The listing builds one solid part. Answer for the finished solid, in the listing's coordinates (mm). A direction names the side the tool comes from. Coordinates: 2 decimals unless noted, no trailing zeros. Loops run counter-clockwise (first coordinate to the right, second up) from the corner with the lowest first, then second, coordinate; pieces in that order, holes last. Notation, with made-up numbers: (-3, 0.5) - (45, 0.5) arc R30 cw to (45, 38.5) - close; hole circle Ø10 at (39.25, -3). An arc over 180 degrees is marked (long way). Return JSON: item names as keys, results as strings. Group by question number.
1. This flat-tipped pin is pushed along its axis until it touches: P1, Ø1, axis at y = -5.5, z = 13, coming from the -X side. Where does it stop, or does it pass through?
2. Which of the six approach directions +Z, -Z, +X, -X, +Y, -Y give full straight-line access (tool end or side, diameter ignored) to faces 4 (the face through (0, 2, 15)), 5 (the face through (17.26, 0.5, 15.18))?
3. Find the intervals of material crossed by line 1 along Z through (x, y) = (29.25, 4); line 2 along Z through (x, y) = (29, -2); line 3 along Z through (x, y) = (29.25, -2.5), in increasing order.
4. Section B-B (z = 2.75) is taken. Write down the section's boundary in (x, y).
5. Section A-A (x = 29.25) is taken. Write down the section's boundary in (y, z), and give its area (3 significant figures).
6. Section D-D (x = 10.5) is taken. Write down the section's boundary in (y, z).
7. The mould has two halves that part along Z. Classify faces 1 (the face through (27.736, 0.098, 3.227)), 2 (the face through (20, 0, 30)), 3 (the face through (40, 0, 15)): pulls with the +Z half, pulls with the -Z half, needs draft (parallel to the pull), parting line crosses it, or undercut.
Autodesk Inventor part; units mm, degrees
ref_plane "YZ Plane" through (0, 0, 0) normal (1, 0, 0) x (0, 1, 0)
ref_plane "XZ Plane" through (0, 0, 0) normal (0, 1, 0) x (-1, 0, 0)
ref_plane "XY Plane" through (0, 0, 0) normal (0, 0, 1) x (1, 0, 0)
sketch "Sketch1" plane through (0, 0, 0) normal (0, 0, 1) x (1, 0, 0)
  line L0 (20, -7) -> (-20, -7)
  line L1 (-20, -7) -> (-20, 7)
  line L2 (-20, 7) -> (20, 7)
  line L3 (20, 7) -> (20, -7)
  line L4 (20, -7) -> (-20, 7) construction
  line L5 (-20, -7) -> (20, 7) construction
  point P0 (0, 0)
  dimension "d0" = 40
  dimension "d1" = 14
extrude "Extrusion1" add sketch "Sketch1" along normal blind 30
sketch "Sketch2" plane through (20, -7, 0) normal (1, 0, 0) x (0, 0, -1)
  point P0 (0, 7)
sketch "Sketch3" plane through (20, -7, 0) normal (1, 0, 0) x (0, 0, -1)
  line L0 (0, 0) -> (-30, 0)
  line L1 (-15, 0) -> (-15, -2)
  arc A0 (-5.7129, 0) -> (-24.2871, 0) centre (-15, -2) ccw
  point P0 (0, 7)
  dimension "d4" = 2
  dimension "d5" = 19
extrude "Extrusion2" cut sketch "Sketch3" against normal blind 35
sketch "Sketch4" plane through (-20, 7, 0) normal (0, 1, 0) x (1, 0, 0)
  point P0 (20, 0)
sketch "Sketch5" plane through (-20, 7, 0) normal (0, 1, 0) x (1, 0, 0)
  line L0 (40, 0) -> (0, 0)
  line L1 (40, -30) -> (0, -30)
  line L2 (0, -30) -> (0, -27.25)
  line L3 (0, 0) -> (0, -30)
  line L4 (0, -27.25) -> (2.75, -27.25)
  circle A0 centre (2.75, -27.25) radius 2
  line L5 (0, 0) -> (0, -2.75)
  line L6 (0, -2.75) -> (2.75, -2.75)
  circle A1 centre (2.75, -2.75) radius 2
  line L7 (2.75, -27.25) -> (10.75, -27.25)
  circle A2 centre (10.75, -27.25) radius 1.5875
  point P0 (20, 0)
  dimension "d11" = 2.75
  dimension "d12" = 2.75
  dimension "d13" = 4
  dimension "d14" = 2.75
  dimension "d15" = 2.75
  dimension "d16" = 4
  dimension "d17" = 8
  dimension "d18" = 3.175
extrude "Extrusion3" cut sketch "Sketch5" against normal blind 100 contours A2
sketch "Sketch6" plane through (-20, 7, 0) normal (0, 1, 0) x (1, 0, 0)
  point P0 (20, 0)
move or copy body "Move Body1" bodies to move or copy 1 copy no translate (-20, 0, 0)
move or copy body "Move Body2" bodies to move or copy 1 copy no translate (-5, 0, 0)
sketch "Sketch8" plane through (0, 0, 0) normal (1, 0, 0) x (0, 1, 0)
  point P0 (0, 0)
move or copy body "Move Body3" bodies to move or copy 1 copy no rotation origin (0, 0, 0) rotation axis (0, 1, 0) rotation angle 180 translate (-10, 0, 0)
move or copy body "Move Body4" bodies to move or copy 1 copy no translate (5, 0, 0)
move or copy body "Move Body5" bodies to move or copy 1 copy no translate (0, 0, 30)
properties part number "Rb oven housing top"
The answers:
{
 "1": {"P1": "stops at x = 35"},
 "2": {"face 4": "+Z, -Z, -X, +Y, -Y", "face 5": "-X, -Y"},
 "3": {"line 1": "z = 0 to 1.16, 4.34 to 30", "line 2": "z = 0 to 1.18, 4.32 to 8.58, 21.42 to 30", "line 3": "z = 0 to 1.16, 4.34 to 8.07, 21.93 to 30"},
 "4": {"outline": "(0, -7) - (27.66, -7) - (27.66, 7) - (0, 7) - close; (30.84, -7) - (40, -7) - (40, 7) - (30.84, 7) - close"},
 "5": {"outline": "(-7, 0) - (7, 0) - (7, 1.16) - (-7, 1.16) - close; (-7, 4.34) - (7, 4.34) - (7, 30) - (-7, 30) - (-7, 24.29) arc R9.5 cw to (-7, 5.71) - close", "area": "272 mm2"},
 "6": {"outline": "(-7, 0) - (7, 0) - (7, 30) - (-7, 30) - (-7, 24.29) arc R9.5 cw to (-7, 5.71) - close"},
 "7": {"face 1": "undercut", "face 2": "pulls with the +Z half", "face 3": "needs draft"}
}
